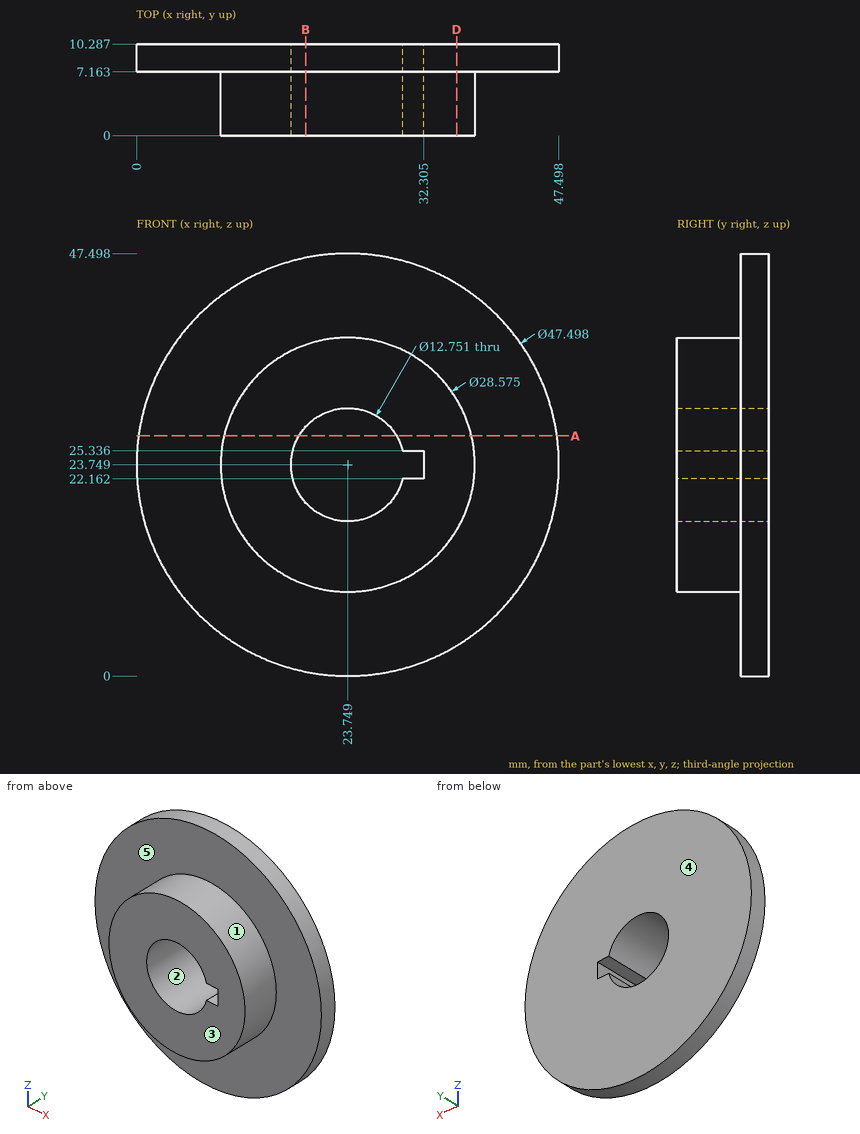
Design review of the part shown in the three views and the two pictorial views. Dimensions are in mm from the part's minimum x, y and z. A direction names the side the tool comes from. Give positions to 0.01 mm unless a question says otherwise; leave off trailing zeros. Write each loop counter-clockwise with the first axis right and the second up, starting at its lowest first coordinate (ties: lowest second). Pieces come first, ordered by that corner, then holes.
Item 1: Machinability: for the marked faces 4 and 5, which of the approach directions +Z, -Z, +X, -X, +Y, -Y give a long, thin tool a straight path to every point of the face, cutting with its end or side? Answer none if there is none.
Item 2: Insertion check: P1, Ø5, axis at y = 2, z = 23.5, coming from the +X side; P2, Ø3.5, axis at y = 2.5, z = 23, coming from the -X side; P3, Ø3, axis at y = 7, z = 30.5, coming from the +X side. Each pin has a flat end and moves straight along its axis. Give the tip position at first contact, or say it passes through.
Item 3: Take a section at B-B (x = 19). Give the boundary of the cut face in (y, z) (1 decimal), and give its area (3 significant figures).
Item 4: Take a section at D-D (x = 36). Give the boundary of the cut face in (y, z) (1 decimal).
Item 5: Take a section at A-A (z = 27). Give the boundary of the cut face in (x, y) (1 decimal).
Item 6: The part is to be moulded in two halves that separate along X. For the marked faces 1, 2 and 3, say which applies: +X half, -X half, draft (parallel to the pull), parting line (faces both ways), or undercut.
Item 7: Wall thickness on probe 1 along X at (y, z) = (6.75, 23.5) (1 decimal); probe 2 along Y at (x, z) = (8.5, 6); probe 3 along Z at (x, y) = (22.5, 1.5) (1 decimal): over which ranges is each line inside the solid? List them lowest first.
Established:
1. face 4: +Z, -Z, +X, -X, +Y
1. face 5: -Y
2. P1: stops at x = 38.04
2. P2: stops at x = 9.46
2. P3: stops at x = 46.91
3. outline: (0, 10.3) - (7.2, 10.3) - (7.2, 0.5) - (10.3, 0.5) - (10.3, 19.5) - (0, 19.5) - close; (0, 28) - (10.3, 28) - (10.3, 47) - (7.2, 47) - (7.2, 37.2) - (0, 37.2) - close
3. area: 251 mm2
4. outline: (0, 16.4) - (7.2, 16.4) - (7.2, 3.4) - (10.3, 3.4) - (10.3, 44.1) - (7.2, 44.1) - (7.2, 31.1) - (0, 31.1) - close
5. outline: (0.2, 7.2) - (9.8, 7.2) - (9.8, 0) - (18.3, 0) - (18.3, 10.3) - (0.2, 10.3) - close; (29.2, 0) - (37.7, 0) - (37.7, 7.2) - (47.3, 7.2) - (47.3, 10.3) - (29.2, 10.3) - close
6. face 1: parting line
6. face 2: undercut
6. face 3: draft
7. probe 1: x = 9.5 to 17.4, 32.3 to 38
7. probe 2: y = 7.16 to 10.29
7. probe 3: z = 9.5 to 17.5, 30 to 38
